CAD build for the part. Positions are in the model's coordinates, mm. Face numbers are marked on the shaded views. A direction names the side the tool comes from. Coordinates: 2 decimals unless noted, no trailing zeros. Write each loop counter-clockwise with the first axis right and the second up, starting at its lowest first coordinate (ties: lowest second). Pieces come first, ordered by that corner, then holes. Notation, with made-up numbers: (6, 47) - (38, 47) arc R33 ccw to (38, 85) - close; hole circle Ø7 at (53, 30). An arc over 180 degrees is marked (long way). Answer in a Markdown table with one row per item. Add a question column.
Q1. Two-plate mould, pull along X, no slides. Class the marked faces 3, 4, 5 and 6: +X half, -X half, draft (parallel to the pull), parting line (faces both ways), or undercut.
Q2. Drill centre lines: line 1 along X through (y, z) = (-15.25, 0); line 2 along Z through (x, y) = (4, -11.5); line 3 along Y through (x, z) = (12, -16.5). Where is each one in solid material? Low to high. Write a range as from..to.
Q3. Band-saw the part on A-A (y = -5). List the corners of the cut face in (x, z), and give its area (3 significant figures).
Q4. Band-saw the part on B-B (z = 21.25). List the corners of the cut face in (x, y), and give its area (3 significant figures).
Q5. Band-saw the part on D-D (x = 4). State how many separate pieces and enclosed holes the cut face has, and give its area (3 significant figures).
Q6. 3-axis set-ups, long thin cutter, end or side, ignore diameter. For the marked faces 1 and 2: which of +Z, -Z, +X, -X, +Y, -Y reach the whole face in a straight line?
Q7. Pin check, flat tips, straight feed: pin 1 (16 mm diameter, centred on x = 0, z = 21.25, fed in from -Y); pin 2 (5 mm diameter, centred on x = 3.5, z = -13, fed in from +Y); pin 3 (5 mm diameter, centred on y = -5, z = 0, fed in from +X). Stop position of each tip, or through.
Q8. Band-saw the part on C-C (y = -15.75). List the corners of the cut face in (x, z), and give its area (3 significant figures).
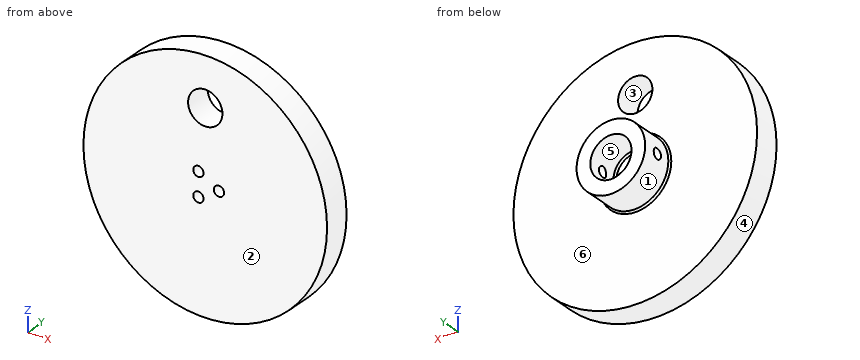
```python
from build123d import *

# Parameters (mm, degrees)
F0_R          = 35.5
F1_DEPTH      = 18
F2_R          = 65
F2_R_2        = 10
F3_DEPTH      = 10
F4_R          = 6
F5_DEPTH      = 10
F6_SIZE       = 0.5
F7_R          = 1.5
F8_DEPTH      = 25
F8_DEPTH_BACK = 25
F9_R          = 5
F10_DEPTH     = 25
F11_SIZE      = 0.5
F12_R         = 1.5
F13_DEPTH     = 20


with BuildPart() as f1:
    # F0 (on Front) → F1 (new body)
    with BuildSketch(Plane.XZ):
        Circle(F0_R)
    extrude(amount=F1_DEPTH)

    # F2 (on face) → F3 (cut)
    with BuildSketch(Plane(origin=(0, 0, 0), x_dir=(-1, 0, 0), z_dir=(0, 1, 0))):
        Circle(F2_R)
        Circle(F2_R_2, mode=Mode.SUBTRACT)
    extrude(amount=-F3_DEPTH, mode=Mode.SUBTRACT)

    # F4 (on face) → F5 (cut)
    with BuildSketch(Plane(origin=(0, 0, 0), x_dir=(-1, 0, 0), z_dir=(0, 1, 0))):
        Circle(F4_R)
    extrude(amount=-F5_DEPTH, mode=Mode.SUBTRACT)

    # F6
    f6_edges = [f1.edges().sort_by_distance(p)[0] for p in [
        (10, -10, 0),
    ]]
    chamfer(f6_edges, length=F6_SIZE)

    # F7 (on Right) → F8 (cut, two sides)
    with BuildSketch(Plane.YZ) as f8_sk:
        with Locations((-5, 0)):
            Circle(F7_R)
    extrude(amount=F8_DEPTH, mode=Mode.SUBTRACT)
    extrude(f8_sk.sketch, amount=-F8_DEPTH_BACK, mode=Mode.SUBTRACT)

    # F9 (on Front) → F10 (cut)
    with BuildSketch(Plane.XZ):
        with Locations((0, 21.25)):
            Circle(F9_R)
    extrude(amount=F10_DEPTH, mode=Mode.SUBTRACT)

    # F11
    f11_edges = [f1.edges().sort_by_distance(p)[0] for p in [
        (6, -10, 0),
    ]]
    chamfer(f11_edges, length=F11_SIZE)

    # F12 (on Front) → F13 (cut)
    with BuildSketch(Plane.XZ):
        with Locations((-2, 3.464102)):
            Circle(F12_R)
        with Locations((-2, -3.464102)):
            Circle(F12_R)
        with Locations((4, 0)):
            Circle(F12_R)
    extrude(amount=F13_DEPTH, mode=Mode.SUBTRACT)


solid = f1.part
```
Checked values:
| question | item | result |
|---|---|---|
| 1 | face 3 | undercut |
| 1 | face 4 | parting line |
| 1 | face 5 | undercut |
| 1 | face 6 | draft |
| 2 | line 1 | x = -35.5..2.5, 5.5..35.5 |
| 2 | line 2 | z = -35.27..-1.5, 1.5..18.25, 24.25..35.27 |
| 2 | line 3 | y = -18..-10 |
| 3 | outline | (-9.89, -1.5) arc R10 ccw to (9.89, -1.5) - (5.81, -1.5) arc R6 cw to (-5.81, -1.5) - close; (-9.89, 1.5) - (-5.81, 1.5) arc R6 cw to (5.81, 1.5) - (9.89, 1.5) arc R10 ccw to start |
| 3 | area | 177 mm² |
| 4 | outline | (-28.44, -18) - (-5, -18) - (-5, -10) - (-28.44, -10) - close; (5, -18) - (28.44, -18) - (28.44, -10) - (5, -10) - close |
| 4 | area | 375 mm² |
| 5 | separate pieces | 3 |
| 5 | enclosed holes | 0 |
| 5 | area | 587 mm² |
| 6 | face 1 | +Y |
| 6 | face 2 | +Z, -Z, +X, -X, -Y |
| 7 | pin 1 | stops at y = -18 |
| 7 | pin 2 | stops at y = -10 |
| 7 | pin 3 | stops at x = 10 |
| 8 | outline | circle Ø71 at (0, 0); hole circle Ø10 at (0, 21.25); hole circle Ø3 at (-2, -3.46); hole circle Ø3 at (-2, 3.46); hole circle Ø3 at (4, 0) |
| 8 | area | 3,860 mm² |
